Autodesk Inventor part; units mm, degrees
ref_plane "YZ Plane" through (0, 0, 0) normal (1, 0, 0) x (0, 1, 0)
ref_plane "XZ Plane" through (0, 0, 0) normal (0, 1, 0) x (-1, 0, 0)
ref_plane "XY Plane" through (0, 0, 0) normal (0, 0, 1) x (1, 0, 0)
sketch "Sketch1" plane through (0, 0, 0) normal (0, 1, 0) x (-1, 0, 0)
  line L0 (0, 0) -> (40, 0)
  line L1 (40, 0) -> (40, -100)
  line L2 (40, -100) -> (0, -100)
  line L3 (0, -100) -> (0, 0)
  dimension "d0" = 100
  dimension "d1" = 40
extrude "Extrusion1" add sketch "Sketch1" along normal blind 5
sketch "Sketch2" plane through (0, 5, 0) normal (0, 1, 0) x (1, 0, 0)
  line L0 (-40, 100) -> (-40, 0)
  line L1 (-40, 89) -> (0, 89) construction
  line L2 (0, 0) -> (0, 100)
  line L3 (0, 100) -> (-40, 100)
  point P0 (-33, 89)
  point P1 (-20, 89)
  point P2 (-7, 89)
  dimension "d4" = 7
  dimension "d5" = 7
  dimension "d6" = 13
  dimension "d7" = 13
  dimension "d8" = 11
hole "Hole1" at (-33, 5, -89) direction (0, -1, 0) diameter 5.5 end through all
hole "Hole2" at (-20, 5, -89) direction (0, -1, 0) diameter 4.134 end through all
sketch "Sketch3" plane through (0, 5, 0) normal (0, 1, 0) x (1, 0, 0)
  line L0 (0, 0) -> (0, 100)
  line L1 (-40, 0) -> (0, 0)
  point P0 (-20, 12)
  point P1 (-20, 37)
  dimension "d23" = 20
  dimension "d24" = 20
  dimension "d25" = 25
  dimension "d26" = 12
hole "Hole3" at (-20, 5, -12) at (-20, 5, -37) direction (0, -1, 0) diameter 8.5 end through all
hole "Hole4" at (-7, 5, -89) direction (0, -1, 0) diameter 5 end through all
properties part number "ER_Verbindungsplatte_Verschraubeinheit"
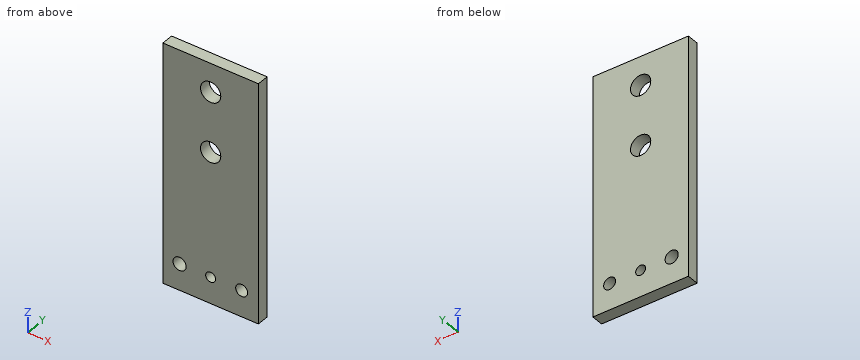
Design review of the part built by this model. Coordinates are the model's own, in mm. Coordinates: 2 decimals unless noted, no trailing zeros. Order: outer loops, then holes, each group sorted by start corner. A loop starts at its lowest first (then second) coordinate and runs counter-clockwise, first axis right, second up. Notation, with made-up numbers: (-25.75, 12) -> (-12.75, 12) arc R14 cw to (-12.75, 34) -> close; hole circle Ø3 at (33.5, 21.5). An arc over 180 degrees is marked (long way). One line per item, written item: value. Start each with the question number.
Q1. Take a section at C-C, the plane x = -33. State the section outline as (y, z) points, then the cut area to 4 significant figures.
Q2. Take a section at D-D, the plane z = -89. State the section outline as (x, y) points.
Q3. Take a section at B-B, the plane y = 1.2. State the section outline as (x, z) points.
Q4. Insertion check: pin 1 Ø2.5 at (x, z) = (-20, -89) entering from -Y (3 decimals); pin 2 Ø8 at (x, z) = (-27, -56.5) entering from -Y. Each pin has a flat end and moves straight along its axis. Give the tip position at first contact, or say it passes through.
Q5. For probe 1 along Z at (x, y) = (-20, 3); probe 2 along X at (y, z) = (3.5, -89); probe 3 along Z at (x, y) = (-33, 4.05), list the stretches that pass through material, from the lowest coordinate up.
Q6. Take a section at A-A, the plane z = -37. State the section outline as (x, y) points, then the cut area to 4 significant figures.
Values follow:
1. outline: (0, -100) -> (5, -100) -> (5, -91.75) -> (0, -91.75) -> close; (0, -86.25) -> (5, -86.25) -> (5, 0) -> (0, 0) -> close
1. area: 472.5 mm2
2. outline: (-40, 0) -> (-35.75, 0) -> (-35.75, 5) -> (-40, 5) -> close; (-30.25, 0) -> (-22.07, 0) -> (-22.07, 5) -> (-30.25, 5) -> close; (-17.93, 0) -> (-9.5, 0) -> (-9.5, 5) -> (-17.93, 5) -> close; (-4.5, 0) -> (0, 0) -> (0, 5) -> (-4.5, 5) -> close
3. outline: (-40, -100) -> (0, -100) -> (0, 0) -> (-40, 0) -> close; hole circle Ø5.5 at (-33, -89); hole circle Ø8.5 at (-20, -37); hole circle Ø8.5 at (-20, -12); hole circle Ø4.13 at (-20, -89); hole circle Ø5 at (-7, -89)
4. pin 1: passes through
4. pin 2: stops at y = 0
5. probe 1: z = -100 to -91.07, -86.93 to -41.25, -32.75 to -16.25, -7.75 to 0
5. probe 2: x = -40 to -35.75, -30.25 to -22.07, -17.93 to -9.5, -4.5 to 0
5. probe 3: z = -100 to -91.75, -86.25 to 0
6. outline: (-40, 0) -> (-24.25, 0) -> (-24.25, 5) -> (-40, 5) -> close; (-15.75, 0) -> (0, 0) -> (0, 5) -> (-15.75, 5) -> close
6. area: 157.5 mm2
